Autodesk Inventor part; units mm, degrees
ref_plane "YZ Plane" through (0, 0, 0) normal (1, 0, 0) x (0, 1, 0)
ref_plane "XZ Plane" through (0, 0, 0) normal (0, 1, 0) x (-1, 0, 0)
ref_plane "XY Plane" through (0, 0, 0) normal (0, 0, 1) x (1, 0, 0)
sketch "Sketch1" plane through (0, 0, 0) normal (0, 0, 1) x (1, 0, 0)
  line L0 (-48.8389, 19.9623) -> (19.1611, 19.9623)
  line L1 (19.1611, 19.9623) -> (19.1611, -15.0377)
  line L2 (19.1611, -15.0377) -> (-48.8389, -15.0377)
  line L3 (-48.8389, -15.0377) -> (-48.8389, 19.9623)
  line L4 (-50.0389, 21.1623) -> (20.3611, 21.1623)
  line L5 (20.3611, 21.1623) -> (20.3611, -16.2377)
  line L6 (20.3611, -16.2377) -> (-50.0389, -16.2377)
  line L7 (-50.0389, -16.2377) -> (-50.0389, 21.1623)
  point P0 (0, 0)
  dimension "d0" = 35
  dimension "d1" = 68
  dimension "d2" = 1.2
  dimension "d3" = 1.2
  dimension "d4" = 1.2
  dimension "d5" = 1.2
extrude "Extrusion1" add sketch "Sketch1" along normal blind 20
sketch "Sketch2" plane through (0, 0, 0) normal (0, 0, -1) x (-1, 0, 0)
  line L0 (-20.3611, 21.1623) -> (50.0389, 21.1623)
  line L1 (50.0389, 21.1623) -> (50.0389, -16.2377)
  line L2 (50.0389, -16.2377) -> (-20.3611, -16.2377)
  line L3 (-20.3611, -16.2377) -> (-20.3611, 21.1623)
  point P0 (0, 0)
extrude "Extrusion2" add sketch "Sketch2" along normal blind 1.2
sketch "Sketch3" plane through (-50.0389, -16.2377, 20) normal (-1, 0, 0) x (0, 0, 1)
  line L0 (-21.2, 0) -> (-21.2, 37.4)
  line L1 (-21.2, 22) -> (-15.2, 22)
  line L2 (-15.2, 22) -> (-15.2, 10)
  line L3 (-15.2, 10) -> (-21.2, 10)
  line L4 (-21.2, 10) -> (-21.2, 22)
  line L5 (0, 0) -> (-21.2, 0)
  point P0 (-20, 16.2377)
  dimension "d10" = 10
  dimension "d11" = 22
  dimension "d12" = 6
extrude "Extrusion3" cut sketch "Sketch3" against normal blind 1.2
sketch "Sketch4" plane through (0, 0, 0) normal (0, 0, 1) x (1, 0, 0)
  line L0 (19.1611, -15.0377) -> (-48.8389, -15.0377)
  line L1 (-48.8389, -15.0377) -> (-48.8389, 19.9623)
  circle A0 centre (-44.8389, 9.9623) radius 2.5
  circle A1 centre (-44.8389, -10.0377) radius 2.5
  circle A2 centre (-0.8389, 9.9623) radius 2.5
  circle A3 centre (-0.8389, -10.0377) radius 2.5
  point P0 (0, 0)
  dimension "d15" = 5
  dimension "d16" = 25
  dimension "d17" = 4
  dimension "d18" = 4
  dimension "d19" = 44
  dimension "d20" = 44
  dimension "d21" = 5
  dimension "d22" = 25
  dimension "d23" = 5
  dimension "d24" = 5
  dimension "d25" = 5
  dimension "d26" = 5
hole "Hole1" at (-44.8389, -10.0377, 0) at (-44.8389, 9.9623, 0) at (-0.8389, 9.9623, 0) at (-0.8389, -10.0377, 0) direction (0, 0, -1) diameter 3 depth 8 tip angle 118
sketch "Sketch5" plane through (0, 0, 20) normal (0, 0, 1) x (1, 0, 0)
  line L0 (-50.0389, 21.1623) -> (-55.0389, 21.1623)
  line L1 (-55.0389, 21.1623) -> (-55.0389, 16.1623)
  line L2 (-55.0389, 16.1623) -> (-50.0389, 16.1623)
  line L3 (-50.0389, 16.1623) -> (-50.0389, 21.1623)
  line L4 (-50.0389, -16.2377) -> (-55.0389, -16.2377)
  line L5 (-55.0389, -16.2377) -> (-55.0389, -11.2377)
  line L6 (-55.0389, -11.2377) -> (-50.0389, -11.2377)
  line L7 (-50.0389, -11.2377) -> (-50.0389, -16.2377)
  line L8 (20.3611, -16.2377) -> (25.3611, -16.2377)
  line L9 (25.3611, -16.2377) -> (25.3611, -11.2377)
  line L10 (25.3611, -11.2377) -> (20.3611, -11.2377)
  line L11 (20.3611, -11.2377) -> (20.3611, -16.2377)
  line L12 (20.3611, 21.1623) -> (25.3611, 21.1623)
  line L13 (25.3611, 21.1623) -> (25.3611, 16.1623)
  line L14 (25.3611, 16.1623) -> (20.3611, 16.1623)
  line L15 (20.3611, 16.1623) -> (20.3611, 21.1623)
  line L16 (20.3611, -16.2377) -> (20.3611, 21.1623)
  point P0 (0, 0)
  dimension "d34" = 5
  dimension "d35" = 5
  dimension "d36" = 5
  dimension "d37" = 5
  dimension "d38" = 5
  dimension "d39" = 5
  dimension "d40" = 5
  dimension "d41" = 5
extrude "Extrusion4" add sketch "Sketch5" against normal blind 21.2
sketch "Sketch6" plane through (20.3611, -11.2377, -1.2) normal (1, 0, 0) x (0, 0, -1)
  line L0 (-21.2, 0) -> (0, 0)
  line L1 (-19.2, 0) -> (-1.2, 0)
  line L2 (-1.2, 0) -> (-1.2, 2)
  line L3 (-1.2, 2) -> (-19.2, 2)
  line L4 (-19.2, 2) -> (-19.2, 0)
  line L5 (-1.2, -3.8) -> (-1.2, 31.2)
  line L6 (-19.2, 4) -> (-1.2, 4)
  line L7 (-1.2, 4) -> (-1.2, 6)
  line L8 (-1.2, 6) -> (-19.2, 6)
  line L9 (-19.2, 6) -> (-19.2, 4)
  line L10 (-19.2, 8) -> (-1.2, 8)
  line L11 (-1.2, 8) -> (-1.2, 10)
  line L12 (-1.2, 10) -> (-19.2, 10)
  line L13 (-19.2, 10) -> (-19.2, 8)
  line L14 (-19.2, 12) -> (-1.2, 12)
  line L15 (-1.2, 12) -> (-1.2, 14)
  line L16 (-1.2, 14) -> (-19.2, 14)
  line L17 (-19.2, 14) -> (-19.2, 12)
  line L18 (-19.2, 16) -> (-1.2, 16)
  line L19 (-1.2, 16) -> (-1.2, 18)
  line L20 (-1.2, 18) -> (-19.2, 18)
  line L21 (-19.2, 18) -> (-19.2, 16)
  line L22 (-19.2, 20) -> (-1.2, 20)
  line L23 (-1.2, 20) -> (-1.2, 22)
  line L24 (-1.2, 22) -> (-19.2, 22)
  line L25 (-19.2, 22) -> (-19.2, 20)
  line L26 (-19.2, 24) -> (-1.2, 24)
  line L27 (-1.2, 24) -> (-1.2, 26)
  line L28 (-1.2, 26) -> (-19.2, 26)
  line L29 (-19.2, 26) -> (-19.2, 24)
  point P0 (-1.2, 11.2377)
  point P1 (-19.2, -2)
  dimension "d44" = 18
  dimension "d45" = 2
  dimension "d46" = 2
  dimension "d47" = 18
  dimension "d48" = 2
  dimension "d49" = 18
  dimension "d50" = 2
  dimension "d51" = 18
  dimension "d52" = 2
  dimension "d53" = 18
  dimension "d54" = 2
  dimension "d55" = 18
  dimension "d56" = 2
  dimension "d57" = 18
  dimension "d58" = 2
extrude "Extrusion5" cut sketch "Sketch6" against normal blind 1.2
sketch "Sketch7" plane through (-55.0389, 21.1623, 20) normal (0, 1, 0) x (1, 0, 0)
  line L0 (74.2, 20) -> (72.2, 20)
  line L1 (72.2, 20) -> (72.2, 2)
  line L2 (72.2, 2) -> (74.2, 2)
  line L3 (74.2, 2) -> (74.2, 20)
  line L4 (70.2, 20) -> (68.2, 20)
  line L5 (68.2, 20) -> (68.2, 2)
  line L6 (68.2, 2) -> (70.2, 2)
  line L7 (70.2, 2) -> (70.2, 20)
  line L8 (66.2, 20) -> (64.2, 20)
  line L9 (64.2, 20) -> (64.2, 2)
  line L10 (64.2, 2) -> (66.2, 2)
  line L11 (66.2, 2) -> (66.2, 20)
  line L12 (62.2, 20) -> (60.2, 20)
  line L13 (60.2, 20) -> (60.2, 2)
  line L14 (60.2, 2) -> (62.2, 2)
  line L15 (62.2, 2) -> (62.2, 20)
  point P0 (55.0389, 20)
  point P1 (76.2, 2)
  dimension "d61" = 2
  dimension "d62" = 18
  dimension "d63" = 2
  dimension "d64" = 2
  dimension "d65" = 18
  dimension "d66" = 2
  dimension "d67" = 18
  dimension "d68" = 2
  dimension "d69" = 18
extrude "Extrusion6" cut sketch "Sketch7" against normal blind 100
sketch "Sketch8" plane through (0, 0, 20) normal (0, 0, 1) x (1, 0, 0)
  line L0 (25.3611, -16.2377) -> (-55.0389, -16.2377)
  line L1 (25.3611, -11.2377) -> (25.3611, -16.2377)
  line L2 (25.3611, 21.1623) -> (25.3611, 16.1623)
  line L3 (25.3611, 16.1623) -> (20.3611, 16.1623)
  line L4 (-55.0389, 21.1623) -> (25.3611, 21.1623)
  line L5 (-55.0389, 21.1623) -> (-55.0389, 16.1623)
  line L6 (-55.0389, -16.2377) -> (-55.0389, -11.2377)
  point P0 (0, 0)
  point P1 (22.8611, -13.7377)
  point P2 (22.8611, 18.6623)
  point P3 (-52.5389, 18.6623)
  point P4 (-52.5389, -13.7377)
  dimension "d72" = 2.5
  dimension "d73" = 2.5
  dimension "d74" = 2.5
  dimension "d75" = 2.5
  dimension "d76" = 2.5
  dimension "d77" = 2.5
  dimension "d78" = 2.5
  dimension "d79" = 2.5
hole "Hole2" at (22.8611, -13.7377, 20) at (22.8611, 18.6623, 20) at (-52.5389, 18.6623, 20) at (-52.5389, -13.7377, 20) direction (0, 0, -1) diameter 2 depth 8 tip angle 118 counterbore diameter 5 counterbore depth 2
properties part number "case body"
Design review of the part built by this model. Coordinates are the model's own, in mm. A direction names the side the tool comes from. Round coordinates to 2 decimals unless told otherwise and drop trailing zeros. Order: outer loops, then holes, each group sorted by start corner. A loop starts at its lowest first (then second) coordinate and runs counter-clockwise, first axis right, second up. Notation, with made-up numbers: (-27.75, 88) - (24.25, 88) arc R27 cw to (24.25, 121) - close; hole circle Ø9 at (-30, 5.25). An arc over 180 degrees is marked (long way). One line per question, with ' | ' between items.
Item 1: Take a section at B-B, the plane z = 6. Give the number of separate pieces and of enclosed holes in the cut face, then the cut area to 3 significant figures.
Checks:
separate pieces: 15 | enclosed holes: 0 | area: 317 mm²
Item 2: Wall thickness on line 1 (X direction, y = 18.5, z = 16.25); line 2 (X direction, y = 20, z = 11.5); line 3 (Y direction, x = 4, z = 12.25): over which ranges is each line inside the solid? List them lowest first. Write a range as [from, to].
Checks:
line 1: [-55.04, -53.53], [-51.55, -48.84], [19.16, 21.87], [23.85, 25.36] | line 2: [-55.04, 5.16], [7.16, 9.16], [11.16, 13.16], [15.16, 17.16], [19.16, 25.36] | line 3: [-16.24, -15.04], [19.96, 21.16]
Item 3: Take a section at C-C, the plane x = -18. Write out the cut boundary in (y, z).
Checks:
outline: (-16.24, -1.2) - (21.16, -1.2) - (21.16, 20) - (19.96, 20) - (19.96, 0) - (-15.04, 0) - (-15.04, 20) - (-16.24, 20) - close
Item 4: Draft analysis for pull direction Y (two halves, no side actions). For faces 4 (the face through (-52.5, 18.5, 11.5)), 5 (the face through (25.361, -14, 10)), state which applies: +Y half, -Y half, draft (parallel to the pull), parting line (faces both ways), or undercut.
Checks:
face 4: undercut | face 5: draft
Item 5: Machinability: for faces 1 (the face through (20.361, 0, 9)), 2 (the face through (22.185, 19.399, 14.958)), 3 (the face through (22, -11.238, 10)), which of the approach directions +Z, -Z, +X, -X, +Y, -Y give a long, thin tool a straight path to every point of the face, cutting with its end or side? Answer none if there is none.
Checks:
face 1: +Z, -Z, +X | face 2: +Z | face 3: +X
Item 6: For P1, Ø3, axis at x = -29.5, y = 2.5, coming from the +Z side; P2, Ø1, axis at y = -1, z = 16, coming from the -X side, all flat-tipped, find the tip position at first contact; note any pin that passes through.
Checks:
P1: z = 0 | P2: x = -50.04
Item 7: Take a section at A-A, the plane y = -0.5. Write out the cut boundary in (x, z), then the cut area to 3 significant figures.
Checks:
outline: (-50.04, 4.8) - (-48.84, 4.8) - (-48.84, 20) - (-50.04, 20) - close; (-48.84, -1.2) - (20.36, -1.2) - (20.36, 20) - (19.16, 20) - (19.16, 0) - (-48.84, 0) - close | area: 125 mm²
